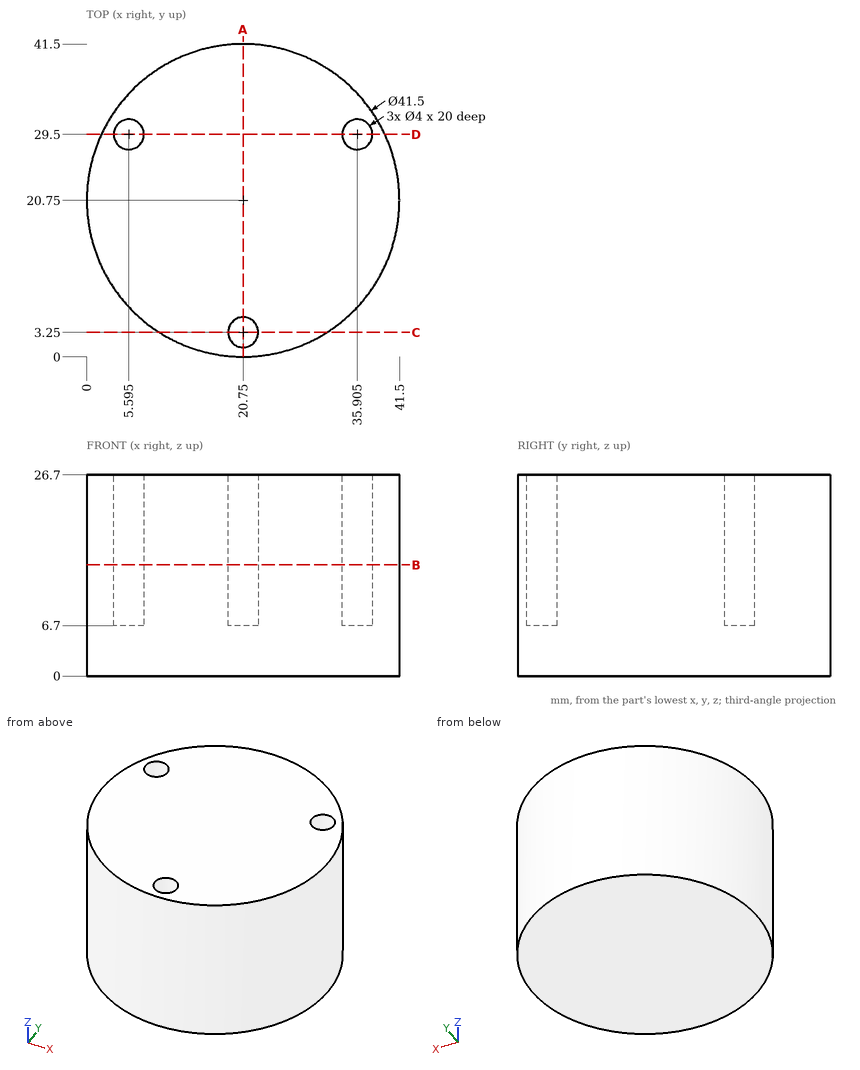
Study the drawing (mm; zero at the part's minimum x, y, z) and answer. Coordinates: 2 decimals unless noted, no trailing zeros. Write each loop counter-clockwise with the first axis right and the second up, starting at its lowest first coordinate (ties: lowest second). Pieces come first, ordered by that corner, then holes. Notation, with made-up numbers: (-11, 67.25) - (30, 67.25) arc R11 ccw to (30, 79.25) - close; hole circle Ø2 at (34.5, -14). An arc over 180 degrees is marked (long way). Answer as a JSON object with one key per item and string values. Group by question number.
1. A cutting plane is placed at C-C (y = 3.25). Determine the outline of the cut face in (x, z).
2. A cutting plane is placed at D-D (y = 29.5). Determine the outline of the cut face in (x, z) (1 decimal), plus the area to 3 significant figures.
3. A cutting plane is placed at A-A (x = 20.75). Determine the outline of the cut face in (y, z), plus the area to 3 significant figures.
4. Consider L1, parallel to Y at x = 20.75, z = 19.75; L2, parallel to Y at x = 5.5, z = 18.5; L3, parallel to X at y = 5, z = 3.25. Determine where each line is inside the solid, lowest interval first. Write a range as [from, to].
5. A cutting plane is placed at B-B (z = 14.75). Give the number of separate pieces and of enclosed holes in the cut face, plus the area to 4 significant figures.
6. Each of these flat-tipped pins is pushed along its axis until it touches: P1, Ø4.5, axis at x = 35.91, y = 29.5, coming from the -Z side; P2, Ø2, axis at x = 6, y = 29.5, coming from the +Z side; P3, Ø2, axis at y = 17.5, z = 5, coming from the +X side; P4, Ø4, axis at y = 6, z = 13.5, coming from the -X side. Where does it stop, or does it pass through?
Worked out:
{
 "1": {"outline": "(9.6, 0) - (31.9, 0) - (31.9, 26.7) - (22.75, 26.7) - (22.75, 6.7) - (18.75, 6.7) - (18.75, 26.7) - (9.6, 26.7) - close"},
 "2": {"outline": "(1.9, 0) - (39.6, 0) - (39.6, 26.7) - (37.9, 26.7) - (37.9, 6.7) - (33.9, 6.7) - (33.9, 26.7) - (7.6, 26.7) - (7.6, 6.7) - (3.6, 6.7) - (3.6, 26.7) - (1.9, 26.7) - close", "area": "845 mm²"},
 "3": {"outline": "(0, 0) - (41.5, 0) - (41.5, 26.7) - (5.25, 26.7) - (5.25, 6.7) - (1.25, 6.7) - (1.25, 26.7) - (0, 26.7) - close", "area": "1,030 mm²"},
 "4": {"L1": "y = [0, 1.25], [5.25, 41.5]", "L2": "y = [6.68, 27.5], [31.5, 34.82]", "L3": "x = [7.24, 34.26]"},
 "5": {"separate pieces": "1", "enclosed holes": "3", "area": "1,315 mm²"},
 "6": {"P1": "stops at z = 0", "P2": "stops at z = 6.7", "P3": "stops at x = 41.38", "P4": "stops at x = 4.38"}
}
